Check sheet for the modelled part. Datum: model origin and axes. Units: mm. A direction names the side the tool comes from. Round coordinates to 2 decimals unless told otherwise and drop trailing zeros. Write each loop counter-clockwise with the first axis right and the second up, starting at its lowest first coordinate (ties: lowest second). Pieces come first, ordered by that corner, then holes. Notation, with made-up numbers: M -26,80.5 L 15,80.5 A20 cw 15,113.5 Z; hole C -2.5,21 d11. An arc over 180 degrees is marked long. Answer in a Markdown table with one row per item.
```python
from build123d import *

# Parameters (mm, degrees)
F2_DEPTH = 55
F1_R     = 78.277093
F3_DEPTH = 60
F5_DEPTH = 60
F6_DEPTH = 53


with BuildPart() as f2:
    # F0 (on Top) → F2 (new body)
    with BuildSketch(Plane.XY):
        Polygon((-4.833426, 28.454347), (-24.831566, 28.454347), (-24.831566, 18.454347), (-4.831566, 18.454347), (-4.831566, 28.454347), align=None)
        Polygon((-24.833426, 28.454347), (-24.831566, 28.454347), (-4.833426, 28.454347), (-3.333426, 30.454347), (-26.333426, 30.454347), align=None)
    extrude(amount=F2_DEPTH)

    # F1 (on Top) → F3 (cut)
    with BuildSketch(Plane.XY):
        with Locations((-14.833426, 107.780978)):
            Circle(F1_R)
    extrude(amount=F3_DEPTH, mode=Mode.SUBTRACT)

    # F4 (on face) → F5 (cut)
    with BuildSketch(Plane.XY.offset(55)):
        with BuildLine():
            ThreePointArc((-13.342683, 21.219841), (-12.598608, 22.103899), (-12.331566, 23.228131))
            ThreePointArc((-12.331566, 23.228131), (-15.943368, 25.467304), (-16.342683, 21.236517))
            Line((-16.342683, 21.236517), (-13.342683, 21.236517))
            Line((-13.342683, 21.236517), (-13.342683, 21.219841))
        make_face()
        with BuildLine():
            Line((-13.342683, 21.236517), (-16.342683, 21.236517))
            ThreePointArc((-16.342683, 21.236517), (-14.845463, 20.72817), (-13.342683, 21.219841))
            Line((-13.342683, 21.219841), (-13.342683, 21.236517))
        make_face()
    extrude(amount=-F5_DEPTH, mode=Mode.SUBTRACT)

    # F4 (on face) → F6 (cut)
    with BuildSketch(Plane.XY.offset(55)):
        with BuildLine():
            ThreePointArc((-13.342683, 21.219841), (-14.845463, 20.72817), (-16.342683, 21.236517))
            Line((-16.342683, 21.236517), (-16.342683, 18.454347))
            Line((-16.342683, 18.454347), (-13.342683, 18.454347))
            Line((-13.342683, 18.454347), (-13.342683, 21.219841))
        make_face()
    extrude(amount=-F6_DEPTH, mode=Mode.SUBTRACT)


solid = f2.part
```
1. Go/stop test with flat-tipped pins: pin 1 (3 mm diameter, centred on x = -17, z = 30.5, fed in from +Y); pin 2 (1.4 mm diameter, centred on y = 19.5, z = 20, fed in from -X); pin 3 (2 mm diameter, centred on x = -15, y = 19.5, fed in from +Z). Record where each tip stops, or that it passes through.
Found:
| item | result |
|---|---|
| pin 1 | stops at y = 29.59 |
| pin 2 | stops at x = -24.83 |
| pin 3 | stops at z = 2 |
2. Section check C-C, the plane y = 21.75. Record the cut outline in (x, z), and give its area (3 significant figures).
Found:
| item | result |
|---|---|
| outline | M -24.83,0 L -16.85,0 L -16.85,55 L -24.83,55 Z; M -12.82,0 L -4.83,0 L -4.83,55 L -12.82,55 Z |
| area | 878 mm2 |
3. Section check B-B, the plane x = -14. Record the cut outline in (y, z), and give its area (3 significant figures).
Found:
| item | result |
|---|---|
| outline | M 18.45,0 L 20.87,0 L 20.87,2 L 18.45,2 Z; M 25.59,0 L 29.51,0 L 29.51,55 L 25.59,55 Z |
| area | 221 mm2 |
4. Access from +Z, -Z, +X, -X, +Y, -Y to the whole of each face (thin tool, end or side, straight path). Record for faces 1 (the face through (-15, 20, 2)), 2 (the face through (-4.832, 23, 27)), 3 (the face through (-12, 24, 0)).
Found:
| item | result |
|---|---|
| face 1 | +Z, -Y |
| face 2 | +Z, -Z, +X, -Y |
| face 3 | -Z, +X, -X, +Y, -Y |
5. Scan lines: L1, parallel to X at y = 23.25, z = 51; L2, parallel to X at y = 20.5, z = 43.5; L3, parallel to X at y = 27.75, z = 16. Record each from-to range of solid material in increasing order.
Found:
| item | result |
|---|---|
| L1 | x = -24.83 to -17.33, -12.33 to -4.83 |
| L2 | x = -24.83 to -16.34, -13.34 to -4.83 |
| L3 | x = -24.83 to -4.83 |
6. Draft check along X on faces 4 (the face through (-12, 24, 55)), 5 (the face through (-4.14, 29.38, 27.12)), 6 (the face through (-24.832, 24, 27)), 7 (the face through (-14.994, 29.504, 27.115)). Enter one of: +X half, -X half, draft (parallel to the pull), parting line (faces both ways), or undercut.
Found:
| item | result |
|---|---|
| face 4 | draft |
| face 5 | +X half |
| face 6 | -X half |
| face 7 | undercut |
7. Section check D-D, the plane x = -22. Record the cut outline in (y, z), and give its area (3 significant figures).
Found:
| item | result |
|---|---|
| outline | M 18.45,0 L 29.83,0 L 29.83,55 L 18.45,55 Z |
| area | 626 mm2 |
